```python
from build123d import *

# Parameters (mm, degrees)
PAD_DEPTH    = 120
SKETCH001_R  = 1.75
PAD001_DEPTH = 3
FILLET_R     = 2


with BuildPart() as part:
    # Sketch → Pad (new body)
    with BuildSketch(Plane.XY):
        Polygon((0, 0), (71.5, 0), (71.5, 11), (69.5, 11), (69.5, 10), (70.5, 10), (70.5, 9), (69.5, 9), (69.5, 3.5), (59.2, 3.5), (59.2, 9), (58.2, 9), (58.2, 10), (59.2, 10), (59.2, 11), (55.2, 11), (55.2, 10), (56.2, 10), (56.2, 9), (55.2, 9), (55.2, 3.5), (44.9, 3.5), (44.9, 9), (43.9, 9), (43.9, 10), (44.9, 10), (44.9, 11), (40.9, 11), (40.9, 10), (41.9, 10), (41.9, 9), (40.9, 9), (40.9, 3.5), (30.6, 3.5), (30.6, 9), (29.6, 9), (29.6, 10), (30.6, 10), (30.6, 11), (26.6, 11), (26.6, 10), (27.6, 10), (27.6, 9), (26.6, 9), (26.6, 3.5), (16.3, 3.5), (16.3, 9), (15.3, 9), (15.3, 10), (16.3, 10), (16.3, 11), (12.3, 11), (12.3, 10), (13.3, 10), (13.3, 9), (12.3, 9), (12.3, 3.5), (2, 3.5), (2, 9), (1, 9), (1, 10), (2, 10), (2, 11), (0, 11), align=None)
    extrude(amount=PAD_DEPTH)

    # Sketch001 → Pad001 (join)
    with BuildSketch(Plane.XZ):
        Polygon((0, 4.994447), (-13, 12.5), (-13, 17.5), (0, 25.005553), align=None)
        with Locations((-9.25, 15)):
            Circle(SKETCH001_R, mode=Mode.SUBTRACT)
        Polygon((0, 65.005553), (-13, 72.5), (-13, 77.5), (0, 84.994447), align=None)
        with Locations((-9.25, 75)):
            Circle(SKETCH001_R, mode=Mode.SUBTRACT)
        Polygon((71.5, 34.994447), (84.5, 42.5), (84.5, 47.5), (71.5, 55.005553), align=None)
        with Locations((80.75, 45)):
            Circle(SKETCH001_R, mode=Mode.SUBTRACT)
        Polygon((71.5, 94.994447), (84.5, 102.5), (84.5, 107.5), (71.5, 115.005553), align=None)
        with Locations((80.75, 105)):
            Circle(SKETCH001_R, mode=Mode.SUBTRACT)
    extrude(amount=-PAD001_DEPTH)

    # Fillet
    fillet_edges = [part.edges().sort_by_distance(p)[0] for p in [
        (2, 3.5, 60),
        (16.3, 3.5, 60),
        (30.6, 3.5, 60),
        (44.9, 3.5, 60),
        (59.2, 3.5, 60),
        (12.3, 3.5, 60),
        (26.6, 3.5, 60),
        (40.9, 3.5, 60),
        (55.2, 3.5, 60),
        (69.5, 3.5, 60),
    ]]
    fillet(fillet_edges, radius=FILLET_R)


solid = part.part
```
Could you check a few things on this model? Use its own coordinates, in mm. A direction names the side the tool comes from. Give positions to 0.01 mm unless a question says otherwise; leave off trailing zeros. Loops run counter-clockwise (first coordinate to the right, second up) from the corner with the lowest first, then second, coordinate; pieces in that order, holes last. Notation, with made-up numbers: (25, 84.25) -> (44, 84.25) arc R5 ccw to (44, 89.25) -> close; hole circle Ø1 at (27.5, 28). An arc over 180 degrees is marked (long way). Put each result on its own line as item: value.
(1) Please list where these lines run through material, in increasing order: probe 1 along Y at (x, z) = (56, 55); probe 2 along X at (y, z) = (5.25, 35.5); probe 3 along Z at (x, y) = (-9.25, 1). Write a range as [from, to].
Computed:
probe 1: [0, 9], [10, 11]
probe 2: [0, 2.02], [12.28, 16.32], [26.58, 30.62], [40.88, 44.92], [55.18, 59.22], [69.48, 71.5]
probe 3: [10.33, 13.25], [16.75, 19.67], [70.34, 73.25], [76.75, 79.66]
(2) For faces 3 (the face through (-5, 3, 75)), 4 (the face through (59.2, 7, 59)), 5 (the face through (76, 3, 105)), 6 (the face through (71.5, 5, 59)), which set-ups out of +Z, -Z, +X, -X, +Y, -Y let a thin tool reach every point of the face, with its end or its side?
Computed:
face 3: +Z, -Z, -X, +Y
face 4: +Z, -Z, +Y
face 5: +Z, -Z, +X, +Y
face 6: +X, +Y
(3) Imagine slicing it at C-C on x = 22.5. Write out the boundary of the cut face in (y, z), plus the area to 3 significant figures.
Computed:
outline: (0, 0) -> (3.5, 0) -> (3.5, 120) -> (0, 120) -> close
area: 420 mm^2
(4) I'm going to push flat-ended pins straight in: pin 1 Ø1 at (y, z) = (7.5, 73) entering from +X; pin 2 Ø3 at (y, z) = (6.5, 31) entering from -X; pin 3 Ø0.5 at (x, z) = (41, 30) entering from -Y; pin 4 Ø4.5 at (x, z) = (-9.25, 75) entering from +Y. Where does each tip first touch, or does it pass through?
Computed:
pin 1: x = 71.5
pin 2: x = 0
pin 3: y = 0
pin 4: y = 3
(5) Imagine slicing it at B-B on x = -9.25. Write out the boundary of the cut face in (y, z), plus the area to 3 significant figures.
Computed:
outline: (0, 10.33) -> (3, 10.33) -> (3, 13.25) -> (0, 13.25) -> close; (0, 16.75) -> (3, 16.75) -> (3, 19.67) -> (0, 19.67) -> close; (0, 70.34) -> (3, 70.34) -> (3, 73.25) -> (0, 73.25) -> close; (0, 76.75) -> (3, 76.75) -> (3, 79.66) -> (0, 79.66) -> close
area: 35.0 mm^2
(6) Imagine slicing it at A-A on y = 1.5. Write out the boundary of the cut face in (x, z).
Computed:
outline: (-13, 12.5) -> (0, 4.99) -> (0, 0) -> (71.5, 0) -> (71.5, 34.99) -> (84.5, 42.5) -> (84.5, 47.5) -> (71.5, 55.01) -> (71.5, 94.99) -> (84.5, 102.5) -> (84.5, 107.5) -> (71.5, 115.01) -> (71.5, 120) -> (0, 120) -> (0, 84.99) -> (-13, 77.5) -> (-13, 72.5) -> (0, 65.01) -> (0, 25.01) -> (-13, 17.5) -> close; hole circle Ø3.5 at (-9.25, 15); hole circle Ø3.5 at (-9.25, 75); hole circle Ø3.5 at (80.75, 45); hole circle Ø3.5 at (80.75, 105)
(7) Thinking about a two-plate mould opening in Z: for faces 1 (the face through (77.909, 1.479, 98.695)), 2 (the face through (55.2, 7, 59)), which applies, pulls with the +Z half, pulls with the -Z half, needs draft (parallel to the pull), parting line crosses it, or undercut?
Computed:
face 1: undercut
face 2: needs draft
